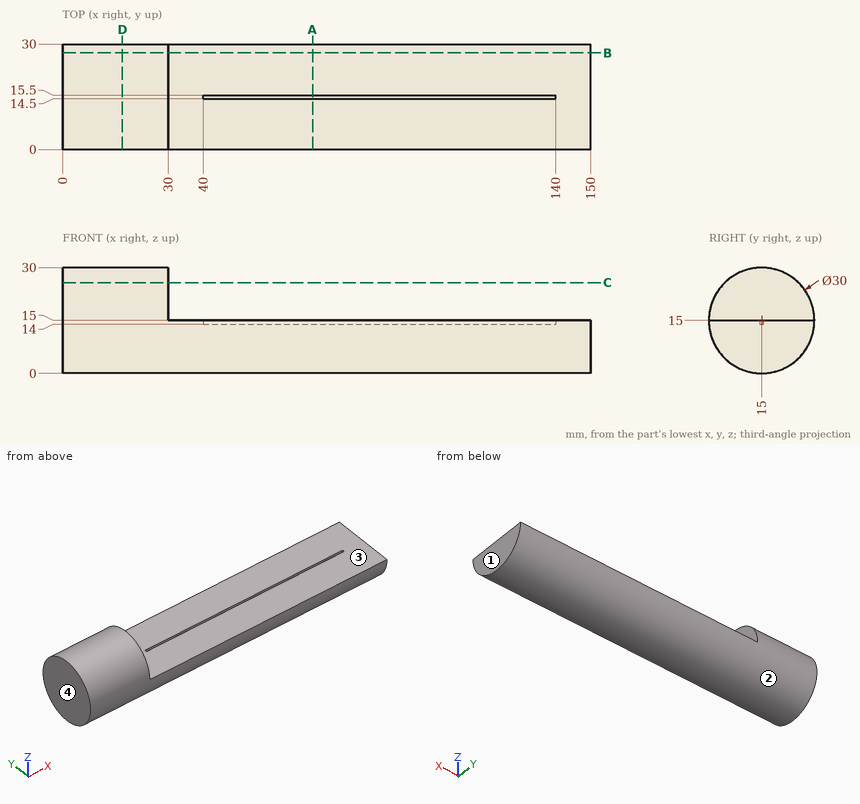
Here's the drawing with two shaded views (mm, measured from the low corner). I have some questions. A direction names the side the tool comes from. Give positions to 0.01 mm unless a question says otherwise; leave off trailing zeros. Loops run counter-clockwise (first coordinate to the right, second up) from the corner with the lowest first, then second, coordinate; pieces in that order, holes last. Notation, with made-up numbers: (25, -35) -> (69, -35) arc R13 ccw to (69, -10) -> close; hole circle Ø6 at (54.5, -37.75). An arc over 180 degrees is marked (long way). Use one line per item in the form item = value.
1) We'd pull the mould along Y, two halves only. Please class the marked faces 1 and 2: released by +Y, released by -Y, zero draft, split by the parting line, or undercut.
Answers:
face_1 = zero draft
face_2 = split by the parting line
2) Will these pins go through, and if not, where does the flat tip stop? pin 1 (8 mm diameter, centred on x = 46, y = 21.5, fed in from -Z); pin 2 (7.5 mm diameter, centred on y = 18, z = 21, fed in from +X); pin 3 (10 mm diameter, centred on x = 121.5, y = 17, fed in from +Z); pin 4 (6 mm diameter, centred on x = 129, z = 20, fed in from +Y).
Answers:
pin_1 = 0.21
pin_2 = 30
pin_3 = 15
pin_4 = through
3) If we section it at A-A (x = 71): Please give me the cut outline in (y, z).
Answers:
outline = (0, 15) arc R15 ccw to (30, 15) -> (15.5, 15) -> (15.5, 14) -> (14.5, 14) -> (14.5, 15) -> close
4) I need wall thicknesses on line 1 along Y through (x, z) = (113, 14.5); line 2 along X through (y, z) = (7.75, 27); line 3 along Z through (x, y) = (63, 9). Which ranges of each line are inside material? Lowest first, please.
Answers:
line_1 = 0.01 to 14.5, 15.5 to 29.99
line_2 = 0 to 30
line_3 = 1.25 to 15
5) If we section it at C-C (z = 25.75): Please give me the cut outline in (x, y).
Answers:
outline = (0, 4.54) -> (30, 4.54) -> (30, 25.46) -> (0, 25.46) -> close
6) If we section it at B-B (y = 27.5): Please give me the cut outline in (x, z), plus the area to 3 significant figures.
Answers:
outline = (0, 6.71) -> (150, 6.71) -> (150, 15) -> (30, 15) -> (30, 23.29) -> (0, 23.29) -> close
area = 1,490 mm²
7) If we section it at D-D (x = 17): Please give me the cut outline in (y, z), plus the area to 3 significant figures.
Answers:
outline = circle Ø30 at (15, 15)
area = 707 mm²
8) For the marked faces 3 and 4, which set-ups out of +Z, -Z, +X, -X, +Y, -Y let a thin tool reach every point of the face, with its end or its side?
Answers:
face_3 = +Z, +X, +Y, -Y
face_4 = +Z, -Z, -X, +Y, -Y
